from build123d import *

# Parameters (mm, degrees)
SKETCH1_R           = 66.675
BOSS_EXTRUDE1_DEPTH = 6.35
CUT_EXTRUDE1_DEPTH  = 95.50626302
CIRPATTERN1_COUNT   = 6
CIRPATTERN1_ANGLE   = 150
CUT_EXTRUDE2_START  = -6.35
CUT_EXTRUDE2_DEPTH  = 6.35


with BuildPart() as part:
    # Sketch1 → Boss-Extrude1 (new body)
    with BuildSketch(Plane.XY):
        Circle(SKETCH1_R)
        Polygon((0, 46.018026219), (-23.00901311, 39.852779738), (-39.852779738, 23.00901311), (-46.018026219, 0), (-39.852779738, -23.00901311), (-23.00901311, -39.852779738), (0, -46.018026219), (23.00901311, -39.852779738), (39.852779738, -23.00901311), (46.018026219, 0), (39.852779738, 23.00901311), (23.00901311, 39.852779738), align=None, mode=Mode.SUBTRACT)
    extrude(amount=-BOSS_EXTRUDE1_DEPTH)

    # Sketch2 → Cut-Extrude1 (cut, through all)
    with BuildSketch(Plane.XY):
        Polygon((43.487619293, -9.443607212), (42.383186664, -13.565405898), (50.84759468, -15.83343719), (50.249360339, -18.066078145), (53.316174837, -18.887828613), (53.914409178, -16.655187658), (57.103896257, -17.509808145), (58.208328886, -13.388009459), (55.018841807, -12.533388972), (55.617076148, -10.300748017), (52.55026165, -9.478997549), (51.952027309, -11.711638504), align=None)
    cut_extrude1 = extrude(amount=-CUT_EXTRUDE1_DEPTH, mode=Mode.SUBTRACT)

    # CirPattern1: Cut-Extrude1 ×6 about axis
    cirpattern1_axis = Axis((0, 0, 0), (0, 0, 1))
    for i in range(1, CIRPATTERN1_COUNT):
        add(cut_extrude1.rotate(cirpattern1_axis, i * CIRPATTERN1_ANGLE / (CIRPATTERN1_COUNT - 1)), mode=Mode.SUBTRACT)

    # Sketch3 → Cut-Extrude2 (cut)
    with BuildSketch(Plane(origin=(0, 0, -6.35), x_dir=(-1, 0, 0), z_dir=(0, 0, -1)).offset(CUT_EXTRUDE2_START)):
        with BuildLine():
            Line((-39.852779738, -23.00901311), (-57.742243797, -33.3375))
            ThreePointArc((-57.742243797, -33.3375), (17.256759832, -64.403104468), (66.675, 0))
            ThreePointArc((66.675, 0), (64.403104468, 17.256759832), (57.742243797, 33.3375))
            Line((57.742243797, 33.3375), (39.852779738, 23.00901311))
            Line((39.852779738, 23.00901311), (46.018026219, 0))
            Line((46.018026219, 0), (39.852779738, -23.00901311))
            Line((39.852779738, -23.00901311), (23.00901311, -39.852779738))
            Line((23.00901311, -39.852779738), (0, -46.018026219))
            Line((0, -46.018026219), (-23.00901311, -39.852779738))
            Line((-23.00901311, -39.852779738), (-39.852779738, -23.00901311))
        make_face()
    extrude(amount=CUT_EXTRUDE2_DEPTH, mode=Mode.SUBTRACT)


solid = part.part
Model file for the job. Use its own axes, mm. A direction names the side the tool comes from. Give positions to 0.01 mm unless a question says otherwise; leave off trailing zeros. Order: outer loops, then holes, each group sorted by start corner. A loop starts at its lowest first (then second) coordinate and runs counter-clockwise, first axis right, second up. Notation, with made-up numbers: M 26,49 L 81,49 A17 ccw 81,81 Z; hole C 60.5,9.5 d4. An arc over 180 degrees is marked long. Put each result on its own line as item: value. Start each with the question number.
(1) Pull direction Y, two halves, no side cores. Call faces 4 (the face through (48.67, -28.1, -3.13)), 5 (the face through (27, 39, -6.35)), 6 (the face through (55.53, 17.09, -3.13)): released by +Y, released by -Y, zero draft, split by the parting line, or undercut.
(2) Band-saw the part on B-B on y = 2.5. Give the cut face in (x, z), then the cut area to 3 significant figures.
(3) Band-saw the part on A-A on y = 48.5. Give the cut face in (x, z), then the cut area to 3 significant figures.
(4) Drill centre lines: L1, parallel to Y at x = 57, z = -5.25; L2, parallel to Y at x = 48, z = -4; L3, parallel to X at y = 39.5, z = -0.25. Where is each one in solid material? Low to high. Write a range as [from, to].
(5) Pin check, flat tips, straight feed: pin 1 Ø1 at (x, y) = (-43, 53.5) entering from -Z; pin 2 Ø1 at (y, z) = (-7.5, -1) entering from -X. Stop position of each tip, or through.
(6) Band-saw the part on C-C on x = -4. Give the cut face in (y, z), then the cut area to 3 significant figures.
(7) Tool access for faces 1 (the face through (51.76, -18.47, -3.13)), 2 (the face through (12.967, 56.636, -3.131)), 3 (the face through (56.591, 12.955, -3.131)): list every direction of +Z, -Z, +X, -X, +Y, -Y with a clear straight run to the whole face (end or side of a thin tool).
Results below:
1. face 4: released by -Y
1. face 5: zero draft
1. face 6: undercut
2. outline: M 45.35,-6.35 L 66.63,-6.35 L 66.63,0 L 45.35,0 Z
2. area: 135 mm2
3. outline: M -45.75,-6.35 L -15.2,-6.35 L -15.2,0 L -45.75,0 Z; M -10.79,-6.35 L 10.79,-6.35 L 10.79,0 L -10.79,0 Z; M 15.2,-6.35 L 45.75,-6.35 L 45.75,0 L 15.2,0 Z
3. area: 525 mm2
4. L1: y = [-32.91, -17.48], [-13.06, 13.06], [17.48, 34.59]
4. L2: y = [-27.71, -15.07], [-10.65, 10.65], [15.07, 46.28]
4. L3: x = [-53.72, -42.52], [-35.75, -23.36], [23.36, 35.75], [42.52, 53.72]
5. pin 1: passes through
5. pin 2: stops at x = 43.87
6. outline: M 44.95,-6.35 L 66.55,-6.35 L 66.55,0 L 44.95,0 Z
6. area: 137 mm2
7. face 1: +Z, -Z
7. face 2: +Z, -Z, -Y
7. face 3: +Z, -Z, -X
